```python
from build123d import *

# Parameters (mm, degrees)
F0_W     = 12.5
F0_H     = 23.2
F0_R     = 5.75
F0_R_2   = 1.5875
F1_DEPTH = 22
F2_DEPTH = 26.25
F3_DEPTH = 28.75


with BuildPart() as f1:
    # F0 (on Top) → F1 (new body)
    with BuildSketch(Plane.XY):
        with Locations((-54.248546, -8.758007)):
            Rectangle(F0_W, F0_H)
        with Locations((-54.248546, -3.834351)):
            Circle(F0_R, mode=Mode.SUBTRACT)
        with Locations((-54.248546, -3.834351)):
            Circle(F0_R)
        with Locations((-54.248546, -3.834351)):
            Circle(F0_R_2, mode=Mode.SUBTRACT)
        with Locations((-54.248546, -3.834351)):
            Circle(F0_R_2)
    extrude(amount=F1_DEPTH)

    # F0 (on Top) → F2 (join)
    with BuildSketch(Plane.XY):
        with Locations((-54.248546, -3.834351)):
            Circle(F0_R)
        with Locations((-54.248546, -3.834351)):
            Circle(F0_R_2, mode=Mode.SUBTRACT)
        with Locations((-54.248546, -3.834351)):
            Circle(F0_R_2)
    extrude(amount=F2_DEPTH)

    # F0 (on Top) → F3 (join)
    with BuildSketch(Plane.XY):
        with Locations((-54.248546, -3.834351)):
            Circle(F0_R_2)
    extrude(amount=F3_DEPTH)


solid = f1.part
```
Input: part model. Units: mm. Frame: model coordinates. A direction names the side the tool comes from. Round coordinates to 2 decimals unless told otherwise and drop trailing zeros. Write each loop counter-clockwise with the first axis right and the second up, starting at its lowest first coordinate (ties: lowest second). Pieces come first, ordered by that corner, then holes. Notation, with made-up numbers: (-19, 17.5) - (-3, 17.5) arc R22 cw to (-3, 45.5) - close; hole circle Ø5 at (7, 28.25). An arc over 180 degrees is marked (long way). Write item = value, one per line.
(1) Material intervals for probe 1 along Z at (x, y) = (-58.5, -1.75); probe 2 along Z at (x, y) = (-58.75, -16); probe 3 along Y at (x, z) = (-57.25, 23.25), sorted ascending.
Geometry check:
probe_1 = 0 to 26.25
probe_2 = 0 to 22
probe_3 = -8.74 to 1.07
(2) Contact query for flat-ended pins moving along their axis: pin 1 Ø6 at (x, y) = (-55, -8.5) entering from +Z; pin 2 Ø2 at (y, z) = (-8, 24) entering from +X. Output: stop coordinate, or through.
Geometry check:
pin_1 = 26.25
pin_2 = -49.45
(3) Section query A-A on x = -49.5. Output: boundary loops of the cut face in (y, z), then the cut area to 3 significant figures.
Geometry check:
outline = (-20.36, 0) - (2.84, 0) - (2.84, 22) - (-0.59, 22) - (-0.59, 26.25) - (-7.08, 26.25) - (-7.08, 22) - (-20.36, 22) - close
area = 538 mm^2
(4) Section query D-D on y = -11.5. Output: boundary loops of the cut face in (x, z).
Geometry check:
outline = (-60.5, 0) - (-48, 0) - (-48, 22) - (-60.5, 22) - close
(5) Access query for faces 1 (the cylindrical face through (-55.835, -3.765, 27.482)), 2 (the flat face through (-54, -20.358, 11)). Directions: +Z, -Z, +X, -X, +Y, -Y. A direction counts if a zero-diameter tool reaches every point of the face in a straight line with its end or side. Return the directions, or none.
Geometry check:
face_1 = +Z
face_2 = +Z, -Z, +X, -X, -Y
(6) Section query C-C on x = -54.5. Output: boundary loops of the cut face in (y, z), then the cut area to 3 significant figures.
Geometry check:
outline = (-20.36, 0) - (2.84, 0) - (2.84, 22) - (1.91, 22) - (1.91, 26.25) - (-2.27, 26.25) - (-2.27, 28.75) - (-5.4, 28.75) - (-5.4, 26.25) - (-9.58, 26.25) - (-9.58, 22) - (-20.36, 22) - close
area = 567 mm^2
(7) Section query B-B on y = -1.5. Output: boundary loops of the cut face in (x, z).
Geometry check:
outline = (-60.5, 0) - (-48, 0) - (-48, 22) - (-48.99, 22) - (-48.99, 26.25) - (-59.5, 26.25) - (-59.5, 22) - (-60.5, 22) - close
